from build123d import *

# Parameters (mm, degrees)
SKETCH_2_W               = 120
SKETCH_2_H               = 62
SKETCH_2_R               = 8.5
SKETCH_2_R_2             = 7.5
SKETCH_2_R_3             = 2.5
EXTRUDE_1_DEPTH          = 10
CUT_EXTRUDE_1_REACH      = 70.272
SKETCH_3_W               = 5
SKETCH_3_H               = 10
PATTERN_LINEAR_1_COUNT   = 3
PATTERN_LINEAR_1_PITCH   = 20
MIRROR_1_COPY_1_REACH    = 70.272
MIRROR_1_COPY_1_SKETCH_W = 5
MIRROR_1_COPY_1_SKETCH_H = 10
MIRROR_1_COPY_2_REACH    = 70.272
MIRROR_1_COPY_2_SKETCH_W = 5
MIRROR_1_COPY_2_SKETCH_H = 10


with BuildPart() as part:
    # 스케치2 → 보스-돌출1 (new body)
    with BuildSketch(Plane.XY):
        Rectangle(SKETCH_2_W, SKETCH_2_H)
        with Locations((12.408275183, -5)):
            Circle(SKETCH_2_R, mode=Mode.SUBTRACT)
        with Locations((-24, 0)):
            Circle(SKETCH_2_R_2, mode=Mode.SUBTRACT)
        with Locations((33.706228335, 9.912987345)):
            Circle(SKETCH_2_R_3, mode=Mode.SUBTRACT)
        with Locations((-8.889677969, -19.912987345)):
            Circle(SKETCH_2_R_3, mode=Mode.SUBTRACT)
    extrude(amount=EXTRUDE_1_DEPTH)

    # 스케치3 → 컷-돌출1 (cut, up to next)
    with BuildSketch(Plane.XY.offset(10), mode=Mode.PRIVATE) as cut_extrude_1_sk1:
        with Locations((-57.5, -26)):
            Rectangle(SKETCH_3_W, SKETCH_3_H)
    cut_extrude_1_tool1 = extrude(cut_extrude_1_sk1.sketch, amount=-CUT_EXTRUDE_1_REACH, mode=Mode.PRIVATE) & part.part
    cut_extrude_1 = cut_extrude_1_tool1.solids().sort_by_distance((-57.5, -26, 10))[0]
    add(cut_extrude_1, mode=Mode.SUBTRACT)

    # 선형 패턴1: 컷-돌출1 ×3
    with Locations(*[(0, i * PATTERN_LINEAR_1_PITCH, 0) for i in range(1, PATTERN_LINEAR_1_COUNT)]):
        add(cut_extrude_1, mode=Mode.SUBTRACT)

    # 대칭 복사1: 컷-돌출1 across plane
    add(cut_extrude_1.mirror(Plane(origin=(0, 0, 0), x_dir=(0, 0, 1), z_dir=(1, 0, 0))), mode=Mode.SUBTRACT)

    # 대칭 복사1 copy 1 sketch → 대칭 복사1 copy 1 (cut, up to next)
    with BuildSketch(Plane(origin=(0, 20, 10), x_dir=(-1, 0, 0), z_dir=(0, 0, 1)), mode=Mode.PRIVATE) as mirror_1_copy_1_sk1:
        with Locations((-57.5, 26)):
            Rectangle(MIRROR_1_COPY_1_SKETCH_W, MIRROR_1_COPY_1_SKETCH_H)
    mirror_1_copy_1_tool1 = extrude(mirror_1_copy_1_sk1.sketch, amount=-MIRROR_1_COPY_1_REACH, mode=Mode.PRIVATE) & part.part
    add(mirror_1_copy_1_tool1.solids().sort_by_distance((57.5, -6, 10))[0], mode=Mode.SUBTRACT)

    # 대칭 복사1 copy 2 sketch → 대칭 복사1 copy 2 (cut, up to next)
    with BuildSketch(Plane(origin=(0, 40, 10), x_dir=(-1, 0, 0), z_dir=(0, 0, 1)), mode=Mode.PRIVATE) as mirror_1_copy_2_sk1:
        with Locations((-57.5, 26)):
            Rectangle(MIRROR_1_COPY_2_SKETCH_W, MIRROR_1_COPY_2_SKETCH_H)
    mirror_1_copy_2_tool1 = extrude(mirror_1_copy_2_sk1.sketch, amount=-MIRROR_1_COPY_2_REACH, mode=Mode.PRIVATE) & part.part
    add(mirror_1_copy_2_tool1.solids().sort_by_distance((57.5, 14, 10))[0], mode=Mode.SUBTRACT)


solid = part.part
Work out the finished part from the listing and answer in its coordinate system (mm). A direction names the side the tool comes from. Coordinates: 2 decimals unless noted, no trailing zeros. Write each loop counter-clockwise with the first axis right and the second up, starting at its lowest first coordinate (ties: lowest second). Pieces come first, ordered by that corner, then holes. Notation, with made-up numbers: M -12.75,-7 L 7.25,-7 A37 ccw 7.25,30 Z; hole C -25.5,27 d7. An arc over 180 degrees is marked long. Write item = value, one per line.
1. Flat-ended cylindrical pins translate along their axes: pin 1 (1.5 mm diameter, centred on x = -56.5, z = 2.5, fed in from -Y); pin 2 (3 mm diameter, centred on y = -6, z = 6, fed in from +X); pin 3 (3 mm diameter, centred on x = 33.71, y = 9.91, fed in from +Z); pin 4 (3 mm diameter, centred on y = 12.5, z = 4.5, fed in from -X). Find the tip coordinate at first contact, or state that the pin passes through.
Solution:
pin_1 = -21
pin_2 = 55
pin_3 = through
pin_4 = -55
2. For faces 4 (the face through (-58, 19, 5)), 5 (the face through (55, -26, 5)), 6 (the face through (-55, -26, 5)), determine the directions among +Z, -Z, +X, -X, +Y, -Y from which every point of the face is accessible in a straight line to the end or side of a thin tool.
Solution:
face_4 = +Z, -Z, -X
face_5 = +Z, -Z, +X, -Y
face_6 = +Z, -Z, -X, -Y
3. The part is cut by section B-B (y = -18.5). Determine the outline of the cut face in (x, z), then the cut area to 3 significant figures.
Solution:
outline = M -60,0 L -10.95,0 L -10.95,10 L -60,10 Z; M -6.83,0 L 60,0 L 60,10 L -6.83,10 Z
area = 1,160 mm2
4. Straight lines are drawn through the part: line 1 (Y direction, x = -24, z = 3.75); line 2 (X direction, y = 18, z = 0.5); line 3 (Y direction, x = -28, z = 4.75). For each, find the intervals that lie inside material, in ascending order. Write a range as from..to.
Solution:
line_1 = -31..-7.5, 7.5..31
line_2 = -55..55
line_3 = -31..-6.34, 6.34..31
5. Determine the mould class of faces 1 (the face through (58, -21, 5)), 2 (the face through (55, -6, 5)), 3 (the face through (3.916, -4.626, 4.93)) for opening direction X: released by +X, released by -X, zero draft, split by the parting line, or undercut.
Solution:
face_1 = zero draft
face_2 = released by +X
face_3 = undercut
6. The part is cut by section A-A (x = -24). Determine the outline of the cut face in (y, z).
Solution:
outline = M -31,0 L -7.5,0 L -7.5,10 L -31,10 Z; M 7.5,0 L 31,0 L 31,10 L 7.5,10 Z
7. The part is cut by section C-C (z = 1.25). Determine the outline of the cut face in (x, y).
Solution:
outline = M -60,-21 L -55,-21 L -55,-31 L 55,-31 L 55,-21 L 60,-21 L 60,-11 L 55,-11 L 55,-1 L 60,-1 L 60,9 L 55,9 L 55,19 L 60,19 L 60,31 L -60,31 L -60,19 L -55,19 L -55,9 L -60,9 L -60,-1 L -55,-1 L -55,-11 L -60,-11 Z; hole C -24,0 d15; hole C -8.89,-19.91 d5; hole C 12.41,-5 d17; hole C 33.71,9.91 d5
8. The part is cut by section D-D (y = -5). Determine the outline of the cut face in (x, z), then the cut area to 3 significant figures.
Solution:
outline = M -55,0 L -29.59,0 L -29.59,10 L -55,10 Z; M -18.41,0 L 3.91,0 L 3.91,10 L -18.41,10 Z; M 20.91,0 L 55,0 L 55,10 L 20.91,10 Z
area = 818 mm2
